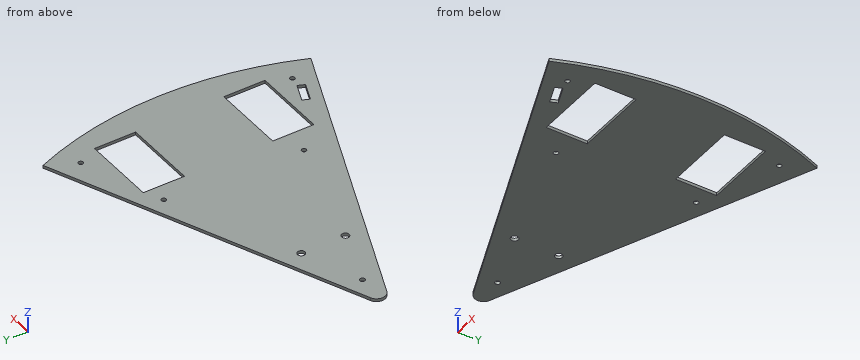
from build123d import *

# Parameters (mm, degrees)
SKETCH_R   = 1.6
SKETCH_R_2 = 1.7
SKETCH_R_3 = 2.5
SKETCH_W   = 50
SKETCH_H   = 28
PAD_DEPTH  = 2
FILLET_R   = 6


with BuildPart() as part:
    # Sketch → Pad (new body)
    with BuildSketch(Plane.XY):
        with BuildLine():
            Line((0, 0), (219.883329, 91.078657))
            ThreePointArc((219.883329, -91.078657), (238, 0), (219.883329, 91.078657))
            Line((0, 0), (219.883329, -91.078657))
        make_face()
        with Locations((155, 52)):
            Circle(SKETCH_R, mode=Mode.SUBTRACT)
        with Locations((150, -40)):
            Circle(SKETCH_R, mode=Mode.SUBTRACT)
        with Locations((210, 72)):
            Circle(SKETCH_R, mode=Mode.SUBTRACT)
        with Locations((210, -72)):
            Circle(SKETCH_R, mode=Mode.SUBTRACT)
        with Locations((30, 0)):
            Circle(SKETCH_R_2, mode=Mode.SUBTRACT)
        with Locations((70, 15)):
            Circle(SKETCH_R_3, mode=Mode.SUBTRACT)
        with Locations((70, -15)):
            Circle(SKETCH_R_3, mode=Mode.SUBTRACT)
        with Locations((192, 44)):
            Rectangle(SKETCH_W, SKETCH_H, mode=Mode.SUBTRACT)
        with Locations((192, -44)):
            Rectangle(SKETCH_W, SKETCH_H, mode=Mode.SUBTRACT)
        Polygon((190, -65), (202.934313, -70.357568), (201.020896, -74.976966), (188.086583, -69.619398), align=None, mode=Mode.SUBTRACT)
    extrude(amount=PAD_DEPTH)

    # Fillet
    fillet_edges = [part.edges().sort_by_distance(p)[0] for p in [
        (0, 0, 1),
    ]]
    fillet(fillet_edges, radius=FILLET_R)


solid = part.part
Could you check a few things on this model? Use its own coordinates, in mm. Round coordinates to 2 decimals unless told otherwise and drop trailing zeros. Write each loop counter-clockwise with the first axis right and the second up, starting at its lowest first coordinate (ties: lowest second). Pieces come first, ordered by that corner, then holes. Notation, with made-up numbers: (30.25, -5.75) - (56.25, -5.75) arc R12 ccw to (56.25, 15.25) - close; hole circle Ø3 at (-34.75, -23.75). An arc over 180 degrees is marked (long way). Use a Markdown table: item, result.
Q1. I want a section at C-C (y = -15). List the corners of the cut face in (x, z) for me.
Output values:
| item | result |
|---|---|
| outline | (36.21, 0) - (67.5, 0) - (67.5, 2) - (36.21, 2) - close; (72.5, 0) - (237.53, 0) - (237.53, 2) - (72.5, 2) - close |
Q2. I want a section at D-D (x = 70). List the corners of the cut face in (y, z) for me, plus the area to 3 significant figures.
Output values:
| item | result |
|---|---|
| outline | (-28.99, 0) - (-17.5, 0) - (-17.5, 2) - (-28.99, 2) - close; (-12.5, 0) - (12.5, 0) - (12.5, 2) - (-12.5, 2) - close; (17.5, 0) - (28.99, 0) - (28.99, 2) - (17.5, 2) - close |
| area | 96.0 mm2 |
Q3. I want a section at B-B (z = 1.7). Count the separate pieces of the cut face and the enclosed holes in it, plus the area to 3 significant figures.
Output values:
| item | result |
|---|---|
| separate pieces | 1 |
| enclosed holes | 10 |
| area | 19,200 mm2 |
Q4. For pin 1 (6 mm diameter, centred on x = 51.5, y = -13, fed in from -Z); pin 2 (0.6 mm diameter, centred on x = 188.5, z = 1, fed in from +Y); pin 3 (1 mm diameter, centred on x = 138, z = 1.5, fed in from +Y); pin 4 (1 mm diameter, centred on x = 180.5, z = 1, fed in from -Y), each with a flat end and sliding along its axis, tell me the tip position at first contact or that it passes through.
Output values:
| item | result |
|---|---|
| pin 1 | z = 0 |
| pin 2 | y = 78.2 |
| pin 3 | y = 57.37 |
| pin 4 | y = -74.97 |
Q5. Please list where these lines run through material, in increasing order: L1, parallel to Y at x = 210, z = 1.15; L2, parallel to Y at x = 183.5, z = 0.25; L3, parallel to X at y = -72, z = 1.3.
Output values:
| item | result |
|---|---|
| L1 | -86.98 to -73.6, -70.4 to -58, -30 to 30, 58 to 70.4, 73.6 to 86.98 |
| L2 | -76.01 to -58, -30 to 30, 58 to 76.01 |
| L3 | 173.82 to 193.83, 202.25 to 208.4, 211.6 to 226.85 |
Q6. I want a section at A-A (x = 195.5). List the corners of the cut face in (y, z) for me, plus the area to 3 significant figures.
Output values:
| item | result |
|---|---|
| outline | (-80.98, 0) - (-72.69, 0) - (-72.69, 2) - (-80.98, 2) - close; (-67.28, 0) - (-58, 0) - (-58, 2) - (-67.28, 2) - close; (-30, 0) - (30, 0) - (30, 2) - (-30, 2) - close; (58, 0) - (80.98, 0) - (80.98, 2) - (58, 2) - close |
| area | 201 mm2 |
